Geometry: final body of the model. Coordinates: model frame, mm. A direction names the side the tool comes from. Give positions to 0.01 mm unless a question says otherwise; leave off trailing zeros. Write each loop counter-clockwise with the first axis right and the second up, starting at its lowest first coordinate (ties: lowest second). Pieces come first, ordered by that corner, then holes. Notation, with made-up numbers: (52.25, 81) -> (62.25, 81) arc R25 cw to (62.25, 116) -> close; hole circle Ø11 at (0.25, 4.5). An arc over 180 degrees is marked (long way). Answer in a Markdown table with one row per item. Add a question column.
Item 1: First-contact query: P1, Ø2.5, axis at x = 0, y = 0, coming from the +Z side; P2, Ø4, axis at y = 10.5, z = 3.5, coming from the -X side; P3, Ø1.5, axis at x = 7.5, z = 5, coming from the -Y side; P4, Ø1.5, axis at y = -1.5, z = 2.5, coming from the -X side. Flat tips, straight axial feed; report the tip coordinate or a pass-through.
Item 2: Access query for faces 4 (the cylindrical face through (-2.377, -10.911, 1.014)), 5 (the flat face through (-6.55, -9.95, 4.43)), 6 (the flat face through (0, 11, 2)). Directions: +Z, -Z, +X, -X, +Y, -Y. A direction counts if a zero-diameter tool reaches every point of the face in a straight line with its end or side. Return the directions, or none.
Item 3: Section query B-B on x = -10.25. Output: boundary loops of the cut face in (y, z), plus the area to 3 significant figures.
Item 4: Section query A-A on y = 0. Output: boundary loops of the cut face in (x, z), plus the area to 3 significant figures.
Item 5: Section query C-C on z = 3.25. State how many separate pieces and enclosed holes the cut face has, plus the area to 3 significant figures.
Item 6: Draft query along Y for faces 1 (the cylindrical face through (7.48, -0.61, 3.45)), 2 (the flat face through (0, -11, 2)), 3 (the cylindrical face through (-7.42, -11.13, 4.37)). Return one class per face: +Y half, -Y half, draft (parallel to the pull), parting line (faces both ways), or undercut.
Item 7: Material intervals for probe 1 along Y at (x, z) = (3, 5); probe 2 along Y at (x, z) = (11, 2); probe 3 along Y at (x, z) = (6, 4.75), sorted ascending. Write a range as from..to.
```python
from build123d import *

# Parameters (mm, degrees)
SKETCH_R        = 13.75
PAD_DEPTH       = 6.8
POCKET_DEPTH    = 4.8
SKETCH002_R     = 1.6
SKETCH002_R_2   = 1.5
POCKET001_DEPTH = 6.801
FILLET_R        = 1


with BuildPart() as part:
    # Sketch → Pad (new body)
    with BuildSketch(Plane.XY):
        Circle(SKETCH_R)
    extrude(amount=PAD_DEPTH)

    # Sketch001 (on Face3 of Pad) → Pocket (cut)
    with BuildSketch(Plane.XY.offset(6.8)):
        with BuildLine():
            ThreePointArc((-6.346376, 9.396063), (-5.339557, 8.083951), (-3.762222, 7.586619))
            Line((-3.762222, 7.586619), (3.762222, 7.586619))
            ThreePointArc((3.762222, 7.586619), (5.339557, 8.083951), (6.346376, 9.396063))
            Line((6.346376, 9.396063), (7.191916, 11.719166))
            ThreePointArc((7.191916, 11.719166), (0, 13.75), (-7.191916, 11.719166))
            Line((-7.191916, 11.719166), (-6.346376, 9.396063))
        make_face()
        with BuildLine():
            Line((-6.346376, -9.396063), (-7.191916, -11.719166))
            ThreePointArc((-7.191916, -11.719166), (0, -13.75), (7.191916, -11.719166))
            Line((6.346376, -9.396063), (7.191916, -11.719166))
            ThreePointArc((6.346376, -9.396063), (5.339557, -8.083951), (3.762222, -7.586619))
            Line((-3.762222, -7.586619), (3.762222, -7.586619))
            ThreePointArc((-3.762222, -7.586619), (-5.339557, -8.083951), (-6.346376, -9.396063))
        make_face()
    extrude(amount=-POCKET_DEPTH, mode=Mode.SUBTRACT)

    # Sketch002 (on Face3 of Pocket) → Pocket001 (cut, through all)
    with BuildSketch(Plane.XY.offset(6.8)):
        with Locations((-10.336619, 3.762222)):
            Circle(SKETCH002_R)
        with Locations((10.336619, 3.762222)):
            Circle(SKETCH002_R)
        with Locations((10.336619, -3.762222)):
            Circle(SKETCH002_R)
        with Locations((-10.336619, -3.762222)):
            Circle(SKETCH002_R)
        with Locations((3.762222, 10.336619)):
            Circle(SKETCH002_R_2)
        with Locations((-3.762222, 10.336619)):
            Circle(SKETCH002_R_2)
        with Locations((-3.762222, -10.336619)):
            Circle(SKETCH002_R_2)
        with Locations((3.762222, -10.336619)):
            Circle(SKETCH002_R_2)
        Circle(SKETCH002_R)
        with Locations((-4.242641, 4.242641)):
            Circle(SKETCH002_R)
        with Locations((4.242641, 4.242641)):
            Circle(SKETCH002_R)
        with Locations((4.242641, -4.242641)):
            Circle(SKETCH002_R)
        with Locations((-4.242641, -4.242641)):
            Circle(SKETCH002_R)
        with Locations((-6, 0)):
            Circle(SKETCH002_R)
        with Locations((6, 0)):
            Circle(SKETCH002_R)
    extrude(amount=-POCKET001_DEPTH, mode=Mode.SUBTRACT)

    # Fillet
    fillet_edges = [part.edges().sort_by_distance(p)[0] for p in [
        (-7.191916, -11.719166, 4.4),
        (7.191916, -11.719166, 4.4),
        (7.191916, 11.719166, 4.4),
        (-7.191916, 11.719166, 4.4),
    ]]
    fillet(fillet_edges, radius=FILLET_R)


solid = part.part
```
Findings below:
| question | item | result |
|---|---|---|
| 1 | P1 | passes through |
| 1 | P2 | stops at x = -10.81 |
| 1 | P3 | stops at y = -11.17 |
| 1 | P4 | stops at x = -13.73 |
| 2 | face 4 | +Z, -Z |
| 2 | face 5 | +Z, -Y |
| 2 | face 6 | +Z, +Y |
| 3 | outline | (-9.17, 0) -> (-5.36, 0) -> (-5.36, 6.8) -> (-9.17, 6.8) -> close; (-2.16, 0) -> (2.16, 0) -> (2.16, 6.8) -> (-2.16, 6.8) -> close; (5.36, 0) -> (9.17, 0) -> (9.17, 6.8) -> (5.36, 6.8) -> close |
| 3 | area | 81.2 mm^2 |
| 4 | outline | (-13.75, 0) -> (-7.6, 0) -> (-7.6, 6.8) -> (-13.75, 6.8) -> close; (-4.4, 0) -> (-1.6, 0) -> (-1.6, 6.8) -> (-4.4, 6.8) -> close; (1.6, 0) -> (4.4, 0) -> (4.4, 6.8) -> (1.6, 6.8) -> close; (7.6, 0) -> (13.75, 0) -> (13.75, 6.8) -> (7.6, 6.8) -> close |
| 4 | area | 122 mm^2 |
| 5 | separate pieces | 1 |
| 5 | enclosed holes | 11 |
| 5 | area | 361 mm^2 |
| 6 | face 1 | undercut |
| 6 | face 2 | draft |
| 6 | face 3 | -Y half |
| 7 | probe 1 | y = -7.59..-5.25, -3.23..3.23, 5.25..7.59 |
| 7 | probe 2 | y = -8.25..-5.22, -2.31..2.31, 5.22..8.25 |
| 7 | probe 3 | y = -8.74..-1.6, 1.6..8.74 |
